Read the model definition and answer for the solid it produces. Units are mm, in the model's axes. Face numbers are marked on the shaded views. A direction names the side the tool comes from. Give positions to 0.01 mm unless a question says otherwise; leave off trailing zeros. Write each loop counter-clockwise with the first axis right and the second up, starting at its lowest first coordinate (ties: lowest second). Pieces come first, ordered by that corner, then holes. Notation, with made-up numbers: M 74,-14 L 116,-14 A11 cw 116,-4 Z; hole C 46,23 d1. An arc over 180 degrees is marked long. Use a Markdown table: item, result. Add a question column.
Item 1: A cutting plane is placed at B-B on x = 48. Determine the outline of the cut face in (y, z), then the cut area to 3 significant figures.
Item 2: Consider probe 1 along Y at (x, z) = (-57.5, 1.1); probe 2 along Y at (x, z) = (-57.5, 2.2); probe 3 along X at (y, z) = (-25, 0.45). Determine where each line is inside the solid, lowest interval first. Write a range as [from, to].
Item 3: A cutting plane is placed at C-C on y = 10.5. Determine the outline of the cut face in (x, z), then the cut area to 3 significant figures.
Item 4: Given P1, Ø1.7, axis at x = -59, y = -26, coming from the -Z side; P2, Ø0.8, axis at x = 1.5, z = 2.5, coming from the -Y side; P3, Ø1.2, axis at y = 4.5, z = 3, coming from the -X side, each flat-ended and moving along its own axis, determine where each tip first touches the part or whether it passes through.
Item 5: For the marked faces 1 and 2, determine the directions among +Z, -Z, +X, -X, +Y, -Y from which every point of the face is accessible in a straight line to the end or side of a thin tool.
Item 6: A cutting plane is placed at A-A on z = 0.7. Determine the outline of the cut face in (x, y), then the cut area to 3 significant figures.
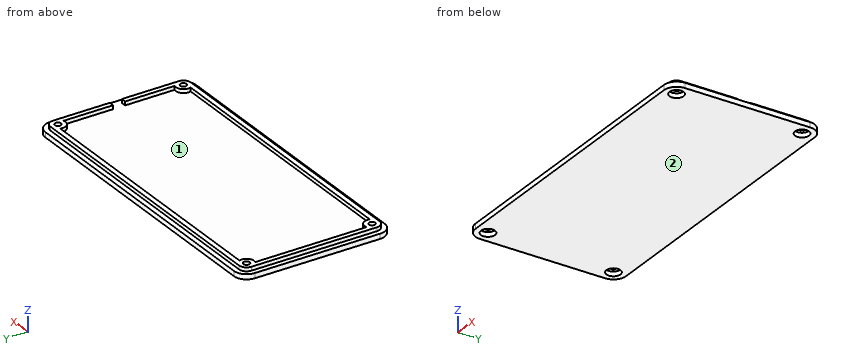
from build123d import *

# Parameters (mm, degrees)
F0_W      = 125
F0_H      = 60
F1_DEPTH  = 2
F2_T      = -2
F3_R      = 5
F4_R      = 1.25
F5_DEPTH  = 10
F6_W      = 117
F6_H      = 52
F7_DEPTH  = 1.5
F8_R      = 3
F9_DEPTH  = 1.5
F10_R     = 1.25
F11_DEPTH = 3.5
F12_R     = 2.8
F13_DEPTH = 1.8
F14_W     = 4.8
F14_H     = 1.5
F15_DEPTH = 2


with BuildPart() as f1:
    # F0 (on Top) → F1 (new body)
    with BuildSketch(Plane.XY):
        Rectangle(F0_W, F0_H)
    extrude(amount=F1_DEPTH)

    # F2
    f2_openings = [f1.faces().sort_by_distance(p)[0] for p in [
        (0, 0, 2),
    ]]
    offset(amount=F2_T, openings=f2_openings)

    # F3
    f3_edges = [f1.edges().sort_by_distance(p)[0] for p in [
        (62.5, -30, 1),
        (62.5, 30, 1),
        (-62.5, 30, 1),
        (-62.5, -30, 1),
    ]]
    fillet(f3_edges, radius=F3_R)

    # F4 (on face) → F5 (cut)
    with BuildSketch(Plane.XY.offset(2)):
        with Locations((-57.5, 25)):
            Circle(F4_R)
        with Locations((-57.5, -25)):
            Circle(F4_R)
        with Locations((57.5, 25)):
            Circle(F4_R)
        with Locations((57.5, -25)):
            Circle(F4_R)
    extrude(amount=F5_DEPTH, mode=Mode.SUBTRACT)

    # F6 (on face) → F7 (join)
    with BuildSketch(Plane.XY.offset(2)):
        with BuildLine():
            ThreePointArc((60.5, 25), (59.62132, 27.12132), (57.5, 28))
            Line((57.5, 28), (-57.5, 28))
            ThreePointArc((-57.5, 28), (-59.62132, 27.12132), (-60.5, 25))
            Line((-60.5, 25), (-60.5, -25))
            ThreePointArc((-60.5, -25), (-59.62132, -27.12132), (-57.5, -28))
            Line((-57.5, -28), (57.5, -28))
            ThreePointArc((57.5, -28), (59.62132, -27.12132), (60.5, -25))
            Line((60.5, -25), (60.5, 25))
        make_face()
        Rectangle(F6_W, F6_H, mode=Mode.SUBTRACT)
    extrude(amount=F7_DEPTH)

    # F8 (on face) → F9 (join)
    with BuildSketch(Plane.XY.offset(2)):
        with Locations((-57.5, 25)):
            Circle(F8_R)
        with Locations((-57.5, -25)):
            Circle(F8_R)
        with Locations((57.5, -25)):
            Circle(F8_R)
        with Locations((57.5, 25)):
            Circle(F8_R)
    extrude(amount=F9_DEPTH)

    # F10 (on face) → F11 (cut, through all)
    with BuildSketch(Plane.XY.offset(3.5)):
        with Locations((57.5, -25)):
            Circle(F10_R)
        with Locations((57.5, 25)):
            Circle(F10_R)
        with Locations((-57.5, 25)):
            Circle(F10_R)
        with Locations((-57.5, -25)):
            Circle(F10_R)
    extrude(amount=-F11_DEPTH, mode=Mode.SUBTRACT)

    # F12 (on face) → F13 (cut)
    with BuildSketch(Plane(origin=(0, 0, 0), x_dir=(1, 0, 0), z_dir=(0, 0, -1))):
        with Locations((-57.5, 25)):
            Circle(F12_R)
        with Locations((57.5, 25)):
            Circle(F12_R)
        with Locations((-57.5, -25)):
            Circle(F12_R)
        with Locations((57.5, -25)):
            Circle(F12_R)
    extrude(amount=-F13_DEPTH, mode=Mode.SUBTRACT)

    # F14 (on face) → F15 (cut, through all)
    with BuildSketch(Plane.YZ.offset(60.5)):
        with Locations((0, 2.75)):
            Rectangle(F14_W, F14_H)
    extrude(amount=-F15_DEPTH, mode=Mode.SUBTRACT)


solid = f1.part
Filled in:
| question | item | result |
|---|---|---|
| 1 | outline | M -30,0 L 30,0 L 30,2 L 28,2 L 28,3.5 L 26,3.5 L 26,2 L -26,2 L -26,3.5 L -28,3.5 L -28,2 L -30,2 Z |
| 1 | area | 126 mm² |
| 2 | probe 1 | [-30, -27.8], [-22.2, 22.2], [27.8, 30] |
| 2 | probe 2 | [-28, -26.25], [-23.75, -22], [22, 23.75], [26.25, 28] |
| 2 | probe 3 | [-62.5, -60.3], [-54.7, 54.7], [60.3, 62.5] |
| 3 | outline | M -62.5,0 L 62.5,0 L 62.5,2 L 60.5,2 L 60.5,3.5 L 58.5,3.5 L 58.5,2 L -58.5,2 L -58.5,3.5 L -60.5,3.5 L -60.5,2 L -62.5,2 Z |
| 3 | area | 256 mm² |
| 4 | P1 | z = 1.8 |
| 4 | P2 | y = -28 |
| 4 | P3 | x = -60.5 |
| 5 | face 1 | +Z |
| 5 | face 2 | -Z, +X, -X, +Y, -Y |
| 6 | outline | M -62.5,-25 A5 ccw -57.5,-30 L 57.5,-30 A5 ccw 62.5,-25 L 62.5,25 A5 ccw 57.5,30 L -57.5,30 A5 ccw -62.5,25 Z; hole C -57.5,-25 d5.6; hole C -57.5,25 d5.6; hole C 57.5,-25 d5.6; hole C 57.5,25 d5.6 |
| 6 | area | 7,380 mm² |
